```python
from build123d import *

# Parameters (mm, degrees)
SKETCH1_W           = 50.8
SKETCH1_H           = 76.2
BOSS_EXTRUDE1_DEPTH = 63.5
FILLET2_RADIUS      = 31.75
FILLET2_LENGTH      = 50.8
SKETCH2_R           = 3.175
BOSS_EXTRUDE2_DEPTH = 6.35
SKETCH3_R           = 3.175
CUT_EXTRUDE1_DEPTH  = 6.35
SKETCH4_W           = 6.35
SKETCH4_H           = 6.35
CUT_EXTRUDE2_DEPTH  = 2.54


with BuildPart() as part:
    # Sketch1 → Boss-Extrude1 (new body)
    with BuildSketch(Plane.XY):
        with Locations((25.4, 38.1)):
            Rectangle(SKETCH1_W, SKETCH1_H)
    extrude(amount=BOSS_EXTRUDE1_DEPTH)

    # Fillet2: full round fillet: the end face becomes a half cylinder, R = half its width
    fillet2_face = Plane((25.4, 0, 31.75), x_dir=(1, 0, 0), z_dir=(0, -1, 0))  # on the end face: x along it, z out of the body
    fillet2_slab = fillet2_face.offset(-FILLET2_RADIUS / 2) * Box(FILLET2_LENGTH, 2 * FILLET2_RADIUS, FILLET2_RADIUS, mode=Mode.PRIVATE)  # the body's end, R deep
    fillet2_round = Plane((25.4, 31.75, 31.75), x_dir=(0, -1, 0), z_dir=(1, 0, 0)) * Cylinder(FILLET2_RADIUS, FILLET2_LENGTH, mode=Mode.PRIVATE)  # its axis R under the face
    add(fillet2_slab - fillet2_round, mode=Mode.SUBTRACT)

    # Sketch2 → Boss-Extrude2 (add)
    with BuildSketch(Plane(origin=(50.8, 0, 0), x_dir=(0, 0, -1), z_dir=(1, 0, 0))):
        with Locations(Location((-31.75, 19.05, 0), (0, 0, 180))):
            Circle(SKETCH2_R)
    boss_extrude2 = extrude(amount=BOSS_EXTRUDE2_DEPTH)

    # Mirror1: Boss-Extrude2 across plane
    add(boss_extrude2.mirror(Plane(origin=(25.4, 0, 0), x_dir=(0, 0, 1), z_dir=(1, 0, 0))))

    # Sketch3 → Cut-Extrude1 (cut)
    with BuildSketch(Plane(origin=(0, 76.2, 0), x_dir=(1, 0, 0), z_dir=(0, 1, 0))):
        with Locations(Location((25.4, -31.75, 0), (0, 0, 270))):
            Circle(SKETCH3_R)
    extrude(amount=-CUT_EXTRUDE1_DEPTH, mode=Mode.SUBTRACT)

    # Sketch4 → Cut-Extrude2 (cut)
    with BuildSketch(Plane(origin=(50.8, 0, 0), x_dir=(0, 0, -1), z_dir=(1, 0, 0))):
        with Locations((-31.75, 73.025)):
            Rectangle(SKETCH4_W, SKETCH4_H)
    extrude(amount=-CUT_EXTRUDE2_DEPTH, mode=Mode.SUBTRACT)


solid = part.part
```
Verification items for the finished model (mm, model axes). A direction names the side the tool comes from. Give positions to 0.01 mm unless a question says otherwise; leave off trailing zeros. Write each loop counter-clockwise with the first axis right and the second up, starting at its lowest first coordinate (ties: lowest second). Pieces come first, ordered by that corner, then holes. Notation, with made-up numbers: M 28,21.25 L 38,21.25 A6 ccw 38,30.25 Z; hole C -0.5,-11 d7. An arc over 180 degrees is marked long. One line per question, with ' | ' between items.
1) Mould release check, pull along Z, two halves, no side actions. Record for faces 1 (the flat face through (25, 54, 63.5)), 2 (the flat face through (50, 73, 28.575)), 3 (the flat face through (50.8, 38, 31)): released by +Z, released by -Z, zero draft, split by the parting line, or undercut.
Result:
face 1: released by +Z | face 2: undercut | face 3: zero draft
2) Gauge pin test, flat ends, axial feed: pin 1 Ø10 at (y, z) = (15.5, 49) entering from +X; pin 2 Ø5.5 at (x, z) = (25.4, 31.75) entering from +Y; pin 3 Ø5 at (y, z) = (67, 45.5) entering from -X. Record the tip position at first contact, or that the pin passes through.
Result:
pin 1: stops at x = 50.8 | pin 2: stops at y = 69.85 | pin 3: stops at x = 0
3) Thickness scan on line 1 along X through (y, z) = (73, 31.75) (3 decimals); line 2 along Y through (x, z) = (36, 32.5); line 3 along X through (y, z) = (6.5, 43). Record the ranges inside material, lowest first. Write a range as [from, to].
Result:
line 1: x = [0, 22.225], [28.575, 48.26] | line 2: y = [0.01, 76.2] | line 3: x = [0, 50.8]
4) Section check A-A on z = 31.75. Enter the section's corners in (x, y) (3 decimals).
Result:
outline: M -6.35,15.875 L 0,15.875 L 0,0 L 50.8,0 L 50.8,15.875 L 57.15,15.875 L 57.15,22.225 L 50.8,22.225 L 50.8,69.85 L 48.26,69.85 L 48.26,76.2 L 28.575,76.2 L 28.575,69.85 L 22.225,69.85 L 22.225,76.2 L 0,76.2 L 0,22.225 L -6.35,22.225 Z
5) Section check C-C on y = 61. Enter the section's corners in (x, z).
Result:
outline: M 0,0 L 50.8,0 L 50.8,63.5 L 0,63.5 Z
6) Set-up check for faces 4 (the cylindrical face through (53.93, 18.91, 28.58)), 5 (the flat face through (50, 69.85, 32)), 6 (the flat face through (25, 69.85, 32)), 7 (the cylindrical face through (-3.13, 18.91, 28.58)): record each of +Z, -Z, +X, -X, +Y, -Y from which the full face is reachable in a straight line by a thin tool's end or side.
Result:
face 4: +X | face 5: +X, +Y | face 6: +Y | face 7: -X
7) Section check D-D on x = 12. Enter the section's corners in (y, z), plus the area to 3 significant figures.
Result:
outline: M 31.75,0 L 76.2,0 L 76.2,63.5 L 31.75,63.5 A31.75 ccw Z | area: 4,410 mm2
8) Section check B-B on x = 25.4. Enter the section's corners in (y, z) (3 decimals), plus the area to 3 significant figures.
Result:
outline: M 31.75,0 L 76.2,0 L 76.2,28.575 L 69.85,28.575 L 69.85,34.925 L 76.2,34.925 L 76.2,63.5 L 31.75,63.5 A31.75 ccw Z | area: 4,370 mm2
